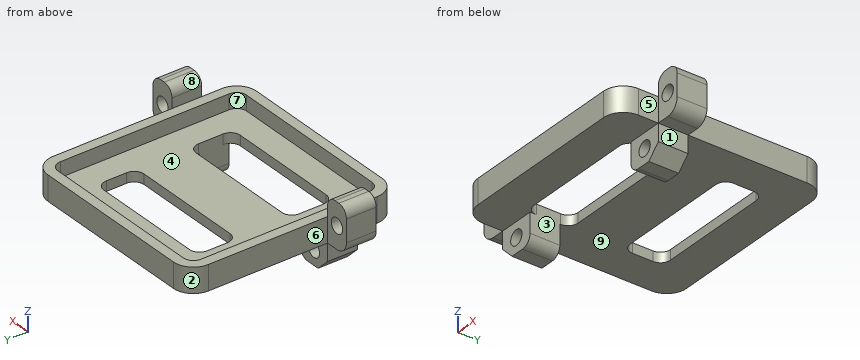
from build123d import *

# Parameters (mm, degrees)
SKETCH1_W           = 41.2
SKETCH1_H           = 42
BOSS_EXTRUDE1_DEPTH = 5
CUT_EXTRUDE1_DEPTH  = 3
FILLET1_R           = 4
CUT_EXTRUDE2_DEPTH  = 2
SKETCH6_W           = 5
SKETCH6_H           = 6
BOSS_EXTRUDE2_DEPTH = 5
SKETCH7_W           = 5
SKETCH7_H           = 6
BOSS_EXTRUDE3_DEPTH = 5
SKETCH8_W           = 7.25
SKETCH8_H           = 6
BOSS_EXTRUDE4_DEPTH = 6
SKETCH9_W           = 7.25
SKETCH9_H           = 6
BOSS_EXTRUDE5_DEPTH = 6
SKETCH13_W          = 5
SKETCH13_H          = 6
BOSS_EXTRUDE6_DEPTH = 4
SKETCH10_R          = 1.5
CUT_EXTRUDE3_DEPTH  = 6
SKETCH12_R          = 1.5
CUT_EXTRUDE4_DEPTH  = 6
FILLET3_R           = 2
FILLET4_R           = 2.5
FILLET6_R           = 2
CUT_EXTRUDE6_START  = -6
CUT_EXTRUDE6_DEPTH  = 6
CUT_EXTRUDE7_START  = -6
CUT_EXTRUDE7_DEPTH  = 6


# Read off the part's stored shape, not the designer's step: Cut-Extrude6, Cut-Extrude7
with BuildPart() as part:
    # Sketch1 → Boss-Extrude1 (new body)
    with BuildSketch(Plane.XY):
        with Locations((20.6, -21)):
            Rectangle(SKETCH1_W, SKETCH1_H)
    extrude(amount=BOSS_EXTRUDE1_DEPTH)

    # Sketch2 → Cut-Extrude1 (cut)
    with BuildSketch(Plane.XY.offset(5)):
        with BuildLine():
            Line((4, -2), (37.2, -2))
            ThreePointArc((37.2, -2), (38.614213562, -2.585786438), (39.2, -4))
            Line((39.2, -4), (39.2, -38))
            ThreePointArc((39.2, -38), (38.614213562, -39.414213562), (37.2, -40))
            Line((37.2, -40), (4, -40))
            ThreePointArc((4, -40), (2.585786438, -39.414213562), (2, -38))
            Line((2, -38), (2, -4))
            ThreePointArc((2, -4), (2.585786438, -2.585786438), (4, -2))
        make_face()
    extrude(amount=-CUT_EXTRUDE1_DEPTH, mode=Mode.SUBTRACT)

    # Fillet1
    fillet1_edges = [part.edges().sort_by_distance(p)[0] for p in [
        (0, 0, 2.5),
        (41.2, 0, 2.5),
        (41.2, -42, 2.5),
        (0, -42, 2.5),
    ]]
    fillet(fillet1_edges, radius=FILLET1_R)

    # Sketch3 → Cut-Extrude2 (cut)
    with BuildSketch(Plane.XY.offset(2)):
        with BuildLine():
            Line((9.25, -7.25), (31.95, -7.25))
            ThreePointArc((31.95, -7.25), (33.364213562, -7.835786438), (33.95, -9.25))
            Line((33.95, -9.25), (33.95, -13.35))
            ThreePointArc((33.95, -13.35), (33.364213562, -14.764213562), (31.95, -15.35))
            Line((31.95, -15.35), (9.25, -15.35))
            ThreePointArc((9.25, -15.35), (7.835786438, -14.764213562), (7.25, -13.35))
            Line((7.25, -13.35), (7.25, -9.25))
            ThreePointArc((7.25, -9.25), (7.835786438, -7.835786438), (9.25, -7.25))
        make_face()
        with BuildLine():
            Line((9.25, -25.85), (31.95, -25.85))
            ThreePointArc((31.95, -25.85), (33.364213562, -26.435786438), (33.95, -27.85))
            Line((33.95, -27.85), (33.95, -32.75))
            ThreePointArc((33.95, -32.75), (33.364213562, -34.164213562), (31.95, -34.75))
            Line((31.95, -34.75), (9.25, -34.75))
            ThreePointArc((9.25, -34.75), (7.835786438, -34.164213562), (7.25, -32.75))
            Line((7.25, -32.75), (7.25, -27.85))
            ThreePointArc((7.25, -27.85), (7.835786438, -26.435786438), (9.25, -25.85))
        make_face()
    extrude(amount=-CUT_EXTRUDE2_DEPTH, mode=Mode.SUBTRACT)

    # Sketch6 → Boss-Extrude2 (add)
    with BuildSketch(Plane(origin=(41.2, 0, 0), x_dir=(0, 0, -1), z_dir=(1, 0, 0))):
        with Locations((-2.5, -31)):
            Rectangle(SKETCH6_W, SKETCH6_H)
    extrude(amount=BOSS_EXTRUDE2_DEPTH)

    # Sketch7 → Boss-Extrude3 (add)
    with BuildSketch(Plane.ZY):
        with Locations((2.5, -31)):
            Rectangle(SKETCH7_W, SKETCH7_H)
    extrude(amount=BOSS_EXTRUDE3_DEPTH)

    # Sketch8 → Boss-Extrude4 (add)
    with BuildSketch(Plane(origin=(0, 0, 0), x_dir=(-1, 0, 0), z_dir=(0, 0, -1))):
        with Locations((-37.575, -31)):
            Rectangle(SKETCH8_W, SKETCH8_H)
    extrude(amount=BOSS_EXTRUDE4_DEPTH)

    # Sketch9 → Boss-Extrude5 (add)
    with BuildSketch(Plane(origin=(0, 0, 0), x_dir=(-1, 0, 0), z_dir=(0, 0, -1))):
        with Locations((-3.625, -31)):
            Rectangle(SKETCH9_W, SKETCH9_H)
    extrude(amount=BOSS_EXTRUDE5_DEPTH)

    # Sketch13 → Boss-Extrude6 (add)
    with BuildSketch(Plane.XY.offset(5)):
        with Locations((43.7, -31)):
            Rectangle(SKETCH13_W, SKETCH13_H)
        with Locations((-2.5, -31)):
            Rectangle(SKETCH13_W, SKETCH13_H)
    extrude(amount=BOSS_EXTRUDE6_DEPTH)

    # Sketch10 → Cut-Extrude3 (cut)
    with BuildSketch(Plane(origin=(0, -28, 0), x_dir=(1, 0, 0), z_dir=(0, 1, 0))):
        with Locations(Location((43.7, -4.5, 0), (0, 0, 180))):
            Circle(SKETCH10_R)
    cut_extrude3 = extrude(amount=-CUT_EXTRUDE3_DEPTH, mode=Mode.SUBTRACT)

    # Mirror1: Cut-Extrude3 across plane
    add(cut_extrude3.mirror(Plane(origin=(20.6, 0, 0), x_dir=(0, 0, 1), z_dir=(1, 0, 0))), mode=Mode.SUBTRACT)

    # Sketch12 → Cut-Extrude4 (cut)
    with BuildSketch(Plane(origin=(0, -28, 0), x_dir=(1, 0, 0), z_dir=(0, 1, 0))):
        with Locations(Location((37.575, 3, 0), (0, 0, 270))):
            Circle(SKETCH12_R)
    cut_extrude4 = extrude(amount=-CUT_EXTRUDE4_DEPTH, mode=Mode.SUBTRACT)

    # Mirror2: Cut-Extrude4 across plane
    add(cut_extrude4.mirror(Plane(origin=(20.6, 0, 0), x_dir=(0, 0, 1), z_dir=(1, 0, 0))), mode=Mode.SUBTRACT)

    # Fillet3
    fillet3_edges = [part.edges().sort_by_distance(p)[0] for p in [
        (33.95, -31, -6),
        (7.25, -31, -6),
    ]]
    fillet(fillet3_edges, radius=FILLET3_R)

    # Fillet4
    fillet4_edges = [part.edges().sort_by_distance(p)[0] for p in [
        (46.2, -31, 0),
        (-5, -31, 0),
    ]]
    fillet(fillet4_edges, radius=FILLET4_R)

    # Fillet6
    fillet6_edges = [part.edges().sort_by_distance(p)[0] for p in [
        (46.2, -31, 9),
        (41.2, -31, 9),
        (0, -31, 9),
        (-5, -31, 9),
    ]]
    fillet(fillet6_edges, radius=FILLET6_R)

    # Cut-Extrude6 outline → Cut-Extrude6 (cut)
    with BuildSketch(Plane(origin=(0, -28, 0), x_dir=(1, 0, 0), z_dir=(0, 1, 0)).offset(CUT_EXTRUDE6_START)):
        Polygon((41.2, 6), (38.7, 6), (41.2, 3.5), align=None)
    extrude(amount=CUT_EXTRUDE6_DEPTH, mode=Mode.SUBTRACT)

    # Cut-Extrude7 outline → Cut-Extrude7 (cut)
    with BuildSketch(Plane(origin=(0, -28, 0), x_dir=(1, 0, 0), z_dir=(0, 1, 0)).offset(CUT_EXTRUDE7_START)):
        Polygon((0, 6), (0, 3.5), (2.5, 6), align=None)
    extrude(amount=CUT_EXTRUDE7_DEPTH, mode=Mode.SUBTRACT)


solid = part.part
Can you work these out from the model? Positions are in its coordinate system, mm. Face numbers are marked on the shaded views. A direction names the side the tool comes from. Give positions to 0.01 mm unless a question says otherwise; leave off trailing zeros. Order: outer loops, then holes, each group sorted by start corner. A loop starts at its lowest first (then second) coordinate and runs counter-clockwise, first axis right, second up. Notation, with made-up numbers: M 60.5,75 L 78.5,75 A24 cw 78.5,88 Z; hole C 25,46 d4. An arc over 180 degrees is marked long. Use a Markdown table: item, result. Add a question column.
Item 1: For the marked faces 5, 6, 7, 8 and 9, which set-ups out of +Z, -Z, +X, -X, +Y, -Y let a thin tool reach every point of the face, with its end or its side?
Item 2: Suppose I cut it at C-C (y = -36.5). List the corners of the cut face in (x, z) for me, then the cut area to 3 significant figures.
Item 3: Will these pins go through, and if not, where does the flat tip stop? pin 1 (10 mm diameter, centred on x = 9, y = -17.5, fed in from +Z); pin 2 (2.5 mm diameter, centred on x = 43, z = 3, fed in from +Y); pin 3 (5.5 mm diameter, centred on x = 44.5, z = 3, fed in from -Y); pin 4 (2.5 mm diameter, centred on x = 43.7, z = 4.5, fed in from -Y).
Item 4: Suppose I cut it at B-B (y = -31). Count the separate pieces of the cut face and the enclosed holes in it, then the cut area to 3 significant figures.
Item 5: We'd pull the mould along Y, two halves only. Please class the marked faces 1, 2, 3 and 4: +Y half, -Y half, draft (parallel to the pull), parting line (faces both ways), or undercut.
Item 6: If I drill on L1, parallel to X at y = -30.5, z = -3 (3 decimals); L2, parallel to Y at x = 13.5, z = 1; L3, parallel to X at y = -10, z = 4.5, over which ranges is the centre line in solid material (lowest first)? Write a range as [from, to].
Item 7: Suppose I cut it at D-D (x = 35). List the corners of the cut face in (y, z) for me, then the cut area to 3 significant figures.
Item 8: Suppose I cut it at A-A (x = 19.5). List the corners of the cut face in (y, z) for me, then the cut area to 3 significant figures.
Answer sheet:
| question | item | result |
|---|---|---|
| 1 | face 5 | +Z, -Z, +X, -Y |
| 1 | face 6 | +Z, -Z, -X, +Y |
| 1 | face 7 | +Z |
| 1 | face 8 | +Z, +Y, -Y |
| 1 | face 9 | -Z, +X, -X, +Y |
| 2 | outline | M 0,0 L 41.2,0 L 41.2,5 L 39.2,5 L 39.2,2 L 2,2 L 2,5 L 0,5 Z |
| 2 | area | 94.4 mm² |
| 3 | pin 1 | stops at z = 2 |
| 3 | pin 2 | stops at y = -28 |
| 3 | pin 3 | stops at y = -34 |
| 3 | pin 4 | passes through |
| 4 | separate pieces | 2 |
| 4 | enclosed holes | 4 |
| 4 | area | 176 mm² |
| 5 | face 1 | draft |
| 5 | face 2 | +Y half |
| 5 | face 3 | undercut |
| 5 | face 4 | undercut |
| 6 | L1 | x = [0, 2.125], [5.125, 7.25], [33.95, 36.075], [39.075, 41.2] |
| 6 | L2 | y = [-42, -34.75], [-25.85, -15.35], [-7.25, 0] |
| 6 | L3 | x = [0, 2], [39.2, 41.2] |
| 7 | outline | M -42,0 L -34,0 L -34,-5.76 L -28,-5.76 L -28,0 L 0,0 L 0,5 L -2,5 L -2,2 L -40,2 L -40,5 L -42,5 Z |
| 7 | area | 131 mm² |
| 8 | outline | M -42,0 L -34.75,0 L -34.75,2 L -40,2 L -40,5 L -42,5 Z; M -25.85,0 L -15.35,0 L -15.35,2 L -25.85,2 Z; M -7.25,0 L 0,0 L 0,5 L -2,5 L -2,2 L -7.25,2 Z |
| 8 | area | 62.0 mm² |
